Input: dimensioned drawing with shaded views. Units: mm. Origin: part minimum x, y, z. A direction names the side the tool comes from. Round coordinates to 2 decimals unless told otherwise and drop trailing zeros. Order: outer loops, then holes, each group sorted by start corner. A loop starts at its lowest first (then second) coordinate and runs counter-clockwise, first axis right, second up. Notation, with made-up numbers: (78.5, -10) - (93.5, -10) arc R26 cw to (93.5, 23) - close; hole circle Ø1 at (-22, -38). An arc over 180 degrees is marked (long way). Return JSON: item names as keys, results as strings. Group by question number.
1) Ray query, line 1 (Y direction, x = 23.21, z = 2.45); line 2 (Y direction, x = 18.5, z = 3.35) (1 decimal); line 3 (Z direction, x = 9, y = 13). Return the intervals inside material, ascending. Write a range as from..to.
2) Contact query for flat-ended pins moving along their axis: P1, Ø1, axis at x = 9, z = 0.5, coming from the +Y side; P2, Ø0.5, axis at x = 19.5, z = 4, coming from the +Y side; P3, Ø6.5, axis at x = 20, y = 3, coming from the +Z side. Output: stop coordinate, or through.
3) Section B-B, the plane y = 19.5. Return loops of the section in (x, z), plus the area to 3 significant figures.
4) Section A-A, the plane x = 15.59. Return loops of the section in (y, z).
5) Section D-D, the plane z = 4.6. Return loops of the section in (x, y).
6) Access query for the marked faces 1, 2 and 3. Directions: +Z, -Z, +X, -X, +Y, -Y. A direction counts if a zero-diameter tool reaches every point of the face in a straight line with its end or side. Return the directions, or none.
7) Section C-C, the plane z = 2.55. Give the number of separate pieces and of enclosed holes in the cut face, plus the area to 3 significant figures.
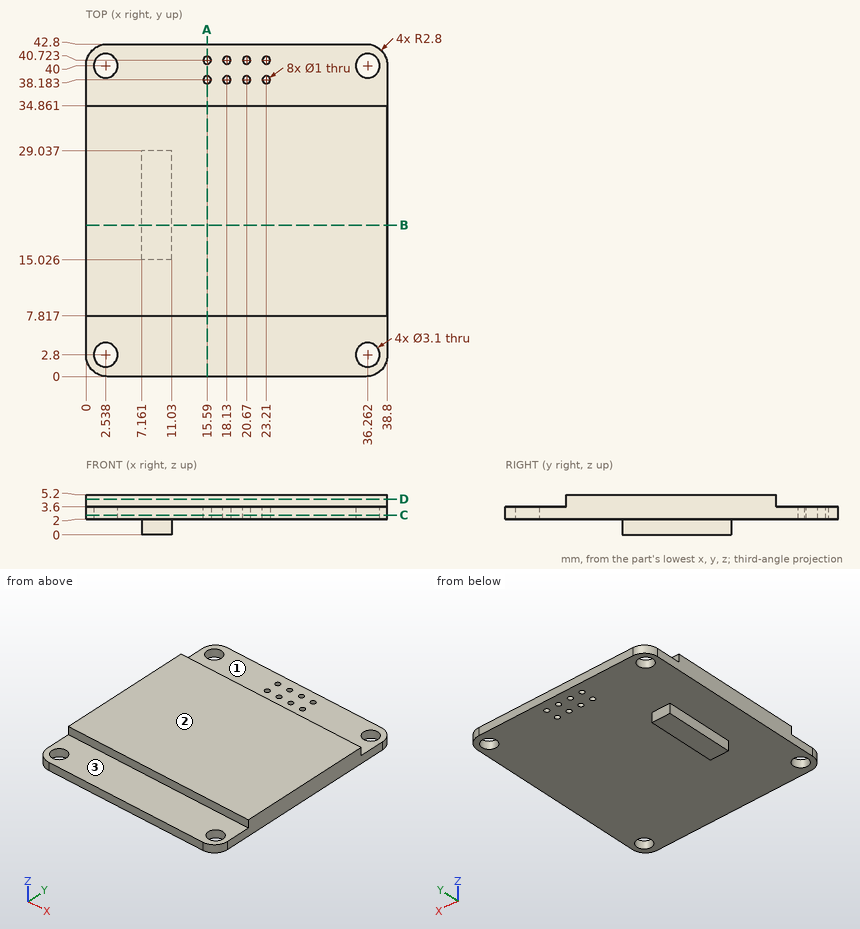
Geometry check:
{
 "1": {"line 1": "0..37.68, 38.68..40.22, 41.22..42.8", "line 2": "0..37.8, 38.5..40.4, 41.1..42.8", "line 3": "2..5.2"},
 "2": {"P1": "y = 29.04", "P2": "y = 34.86", "P3": "z = 3.6"},
 "3": {"outline": "(0, 2) - (7.16, 2) - (7.16, 0) - (11.03, 0) - (11.03, 2) - (38.8, 2) - (38.8, 5.2) - (0, 5.2) - close", "area": "132 mm2"},
 "4": {"outline": "(0, 2) - (37.68, 2) - (37.68, 3.6) - (34.86, 3.6) - (34.86, 5.2) - (7.82, 5.2) - (7.82, 3.6) - (0, 3.6) - close; (38.68, 2) - (40.22, 2) - (40.22, 3.6) - (38.68, 3.6) - close; (41.22, 2) - (42.8, 2) - (42.8, 3.6) - (41.22, 3.6) - close"},
 "5": {"outline": "(0, 7.82) - (38.8, 7.82) - (38.8, 34.86) - (0, 34.86) - close"},
 "6": {"face 1": "+Z, +X, -X, +Y", "face 2": "+Z, +X, -X, +Y, -Y", "face 3": "+Z, +X, -X, -Y"},
 "7": {"separate pieces": "1", "enclosed holes": "12", "area": "1,620 mm2"}
}
